The model under review builds one solid part; all positions refer to its coordinate system, in mm. A direction names the side the tool comes from. Coordinates: 2 decimals unless noted, no trailing zeros. Write each loop counter-clockwise with the first axis right and the second up, starting at its lowest first coordinate (ties: lowest second). Pieces come first, ordered by that corner, then holes. Notation, with made-up numbers: M -7,28.25 L 33,28.25 A12 ccw 33,37.25 Z; hole C 63.25,74 d3. An arc over 180 degrees is marked long. Answer as a JSON object with one key per item and string values.
```python
from build123d import *

# Parameters (mm, degrees)
SKETCH1_W           = 127
SKETCH1_H           = 6.35
BOSS_EXTRUDE1_DEPTH = 63.5
SKETCH2_W           = 127
SKETCH2_H           = 6.35
BOSS_EXTRUDE2_DEPTH = 8.89
CUT_EXTRUDE1_DEPTH  = 64.5


with BuildPart() as part:
    # Sketch1 → Boss-Extrude1 (new body)
    with BuildSketch(Plane.XY):
        Rectangle(SKETCH1_W, SKETCH1_H)
    extrude(amount=-BOSS_EXTRUDE1_DEPTH)

    # Sketch2 → Boss-Extrude2 (add)
    with BuildSketch(Plane(origin=(0, 3.175, 0), x_dir=(1, 0, 0), z_dir=(0, 1, 0))):
        with Locations((0, 60.325)):
            Rectangle(SKETCH2_W, SKETCH2_H)
        with Locations((0, 3.175)):
            Rectangle(SKETCH2_W, SKETCH2_H)
    extrude(amount=BOSS_EXTRUDE2_DEPTH)

    # Sketch3 → Cut-Extrude1 (cut, through all)
    with BuildSketch(Plane.XY):
        Polygon((63.5, -3.175), (30.817714531, 12.065), (41.55221838, 35.085217791), (74.234503848, 19.845217791), align=None)
    extrude(amount=-CUT_EXTRUDE1_DEPTH, mode=Mode.SUBTRACT)


solid = part.part
```
(1) Add section D-D on x = 44.5. Give the boundary of the cut face in (y, z) (3 decimals).
Results list:
{"outline": "M -3.175,-63.5 L 5.685,-63.5 L 5.685,-57.15 L 3.175,-57.15 L 3.175,-6.35 L 5.685,-6.35 L 5.685,0 L -3.175,0 Z"}
(2) Draft analysis for pull direction Z (two halves, no side actions). For faces 1 (the face through (-17, 12.065, -60)), 2 (the face through (-8, 8, -6.35)), 3 (the face through (-15, 4, -63.5)), state which applies: released by +Z, released by -Z, zero draft, split by the parting line, or undercut.
Results list:
{"face 1": "zero draft", "face 2": "undercut", "face 3": "released by -Z"}
(3) For pin 1 Ø5 at (y, z) = (5.5, -24.5) entering from +X; pin 2 Ø5 at (y, z) = (3.5, -18.5) entering from +X, all flat-tipped, find the tip position at first contact; note any pin that passes through.
Results list:
{"pin 1": "x = 50.26", "pin 2": "x = 54.55"}
(4) For faces 4 (the face through (-8, 3.175, -31)), 5 (the face through (-17, 12.065, -3)), list the 3-axis set-ups (+Z, -Z, +X, -X, +Y, -Y) from which the entire face can be reached by the end or side of a thin tool; tool diameter is ignored.
Results list:
{"face 4": "+X, -X, +Y", "face 5": "+Z, -Z, +X, -X, +Y"}
(5) Add section A-A on y = 9.5. Give the boundary of the cut face in (x, z), and give its area (3 significant figures).
Results list:
{"outline": "M -63.5,-63.5 L 36.32,-63.5 L 36.32,-57.15 L -63.5,-57.15 Z; M -63.5,-6.35 L 36.32,-6.35 L 36.32,0 L -63.5,0 Z", "area": "1,270 mm²"}
(6) Add section C-C on z = -35.5. Give the boundary of the cut face in (x, y) (3 decimals).
Results list:
{"outline": "M -63.5,-3.175 L 63.5,-3.175 L 49.882,3.175 L -63.5,3.175 Z"}
(7) Add section B-B on x = -50. Give the boundary of the cut face in (y, z) (3 decimals).
Results list:
{"outline": "M -3.175,-63.5 L 12.065,-63.5 L 12.065,-57.15 L 3.175,-57.15 L 3.175,-6.35 L 12.065,-6.35 L 12.065,0 L -3.175,0 Z"}
(8) Wall thickness on line 1 along Z through (x, y) = (-26.5, 7.5); line 2 along Y through (x, z) = (44, -38.5) (3 decimals); line 3 along X through (y, z) = (-1.5, -36): over which ranges is each line inside the solid? List them lowest first. Write a range as from..to.
Results list:
{"line 1": "-63.5..-57.15, -6.35..0", "line 2": "-3.175..3.175", "line 3": "-63.5..59.91"}
